Autodesk Inventor part; units mm, degrees
ref_plane "YZ Plane" through (0, 0, 0) normal (1, 0, 0) x (0, 1, 0)
ref_plane "XZ Plane" through (0, 0, 0) normal (0, 1, 0) x (-1, 0, 0)
ref_plane "XY Plane" through (0, 0, 0) normal (0, 0, 1) x (1, 0, 0)
sketch "Sketch1" plane through (0, 0, 0) normal (0, 1, 0) x (-1, 0, 0)
  line L0 (-10.795, 10.795) -> (10.795, 10.795)
  line L1 (10.795, 10.795) -> (10.795, -10.795)
  line L2 (-10.795, -10.795) -> (-10.795, 10.795)
  circle A0 centre (5.6576, -5.6576) radius 1.9304
  circle A1 centre (6.9088, 6.9088) radius 1.9304
  circle A2 centre (-5.6576, 5.6576) radius 1.9304
  circle A3 centre (-6.9088, -6.9148) radius 1.9304
  line L3 (-5.715, -10.795) -> (-5.715, -20.574)
  line L4 (-5.715, -20.574) -> (6.985, -20.574)
  line L5 (6.985, -20.574) -> (6.985, -10.795)
  line L6 (10.795, -10.795) -> (6.985, -10.795)
  line L7 (-5.715, -10.795) -> (-10.795, -10.795)
  point P0 (0, 0)
  dimension "d2" = 10.795
  dimension "d3" = 10.795
  dimension "d4" = 3.8608
  dimension "d5" = 5.6576
  dimension "d6" = 5.6576
  dimension "d7" = 3.8608
  dimension "d8" = 6.9088
  dimension "d9" = 6.9088
  dimension "d10" = 3.8608
  dimension "d11" = 5.6576
  dimension "d12" = 5.6576
  dimension "d13" = 3.8608
  dimension "d14" = 12.7
  dimension "d16" = 6.985
  dimension "d45" = 10.795
  dimension "d46" = 10.795
  dimension "d47" = 10.795
extrude "Extrusion1" add sketch "Sketch1" along normal blind 6.985
sketch "Sketch2" plane through (-6.985, 0, -20.574) normal (-1, 0, 0) x (0, 0, 1)
  circle A0 centre (5.08, 3.4925) radius 4.6609 construction
  line L0 (9.779, 0) -> (0, 0)
  line L1 (0, 0) -> (0, 6.985)
  line L2 (9.7409, 3.4925) -> (7.4105, -0.544)
  line L3 (7.4105, -0.544) -> (2.7496, -0.544)
  line L4 (2.7496, -0.544) -> (0.4191, 3.4925)
  line L5 (0.4191, 3.4925) -> (2.7495, 7.529)
  line L6 (2.7495, 7.529) -> (7.4104, 7.529)
  line L7 (7.4104, 7.529) -> (9.7409, 3.4925)
  point P0 (20.574, 0)
  dimension "d19" = 9.3218
  dimension "d20" = 3.4925
  dimension "d21" = 5.08
extrude "Extrusion2" cut sketch "Sketch2" against normal blind 3.81
sketch "Sketch3" plane through (5.715, 0, -10.795) normal (1, 0, 0) x (0, 0, -1)
  circle A0 centre (4.699, 3.4925) radius 1.9304
  line L0 (9.779, 0) -> (9.779, 6.985)
  line L1 (0, 6.985) -> (9.779, 6.985)
  point P0 (-10.795, 0)
  dimension "d24" = 3.8608
  dimension "d25" = 5.08
  dimension "d26" = 3.4925
extrude "Extrusion3" cut sketch "Sketch3" against normal through all
sketch "Sketch4" plane through (0, 6.985, 0) normal (0, 1, 0) x (1, 0, 0)
  circle A0 centre (0, 0) radius 4
  dimension "d29" = 8
extrude "Extrusion4" add sketch "Sketch4" along normal blind 12.7
sketch "Sketch5" plane through (0, 19.685, 0) normal (0, 1, 0) x (1, 0, 0)
  arc A0 (2.0472, -2.5908) -> (-2.0472, -2.5908) centre (0, 0) ccw
  line L0 (-2.0472, -2.5908) -> (2.0472, -2.5908)
  dimension "d32" = 6.604
  dimension "d33" = 2.5908
fillet "Fillet1" radius 3.3782 4 edges at (10.795, 3.4925, 10.795) (10.795, 3.4925, -10.795) (-10.795, 3.4925, 10.795) (-10.795, 3.4925, -10.795)
extrude "Extrusion5" cut sketch "Sketch5" against normal through all
sketch "Sketch6" plane through (0, 19.685, 0) normal (0, 1, 0) x (1, 0, 0)
  line L0 (-6.985, 20.574) -> (5.715, 20.574)
  line L1 (0.635, 0) -> (0.635, 20.574)
  line L2 (0.635, 20.574) -> (-0.635, 20.574)
  line L3 (-0.635, 20.574) -> (-0.635, 0)
  line L4 (-0.635, -20.574) -> (0.635, 20.574) construction
  line L5 (0.635, -20.574) -> (-0.635, 20.574) construction
  line L6 (-0.635, 0) -> (0.635, 0)
  point P0 (0, 0)
  dimension "d37" = 1.27
extrude "Extrusion6" cut sketch "Sketch6" against normal through all
sketch "Sketch7" plane through (0, 0, 0) normal (0, -1, 0) x (1, 0, 0)
  circle A0 centre (-5.6576, -5.6576) radius 1.9304
  circle A1 centre (-5.6576, -5.6576) radius 4.6609 construction
  circle A2 centre (5.6576, 5.6576) radius 1.9304
  circle A3 centre (5.6576, 5.6576) radius 4.6609 construction
  line L0 (-5.6576, -0.9967) -> (-1.6211, -3.3271)
  line L1 (-1.6211, -3.3271) -> (-1.6211, -7.988)
  line L2 (-1.6211, -7.988) -> (-5.6576, -10.3185)
  line L3 (-5.6576, -10.3185) -> (-9.694, -7.988)
  line L4 (-9.694, -7.988) -> (-9.694, -3.3271)
  line L5 (-9.694, -3.3271) -> (-5.6576, -0.9967)
  line L6 (5.6576, 0.9967) -> (1.6211, 3.3271)
  line L7 (1.6211, 3.3271) -> (1.6211, 7.988)
  line L8 (1.6211, 7.988) -> (5.6576, 10.3185)
  line L9 (5.6576, 10.3185) -> (9.694, 7.988)
  line L10 (9.694, 7.988) -> (9.694, 3.3271)
  line L11 (9.694, 3.3271) -> (5.6576, 0.9967)
  point P0 (0, 0)
  dimension "d40" = 9.3218
  dimension "d41" = 9.3218
extrude "Extrusion7" cut sketch "Sketch7" against normal blind 4.3688
fillet "Fillet2" radius 1.27 1 edges at (5.715, 3.4925, -20.574)
properties part number "clamping hub .25 in to 8mm hub"
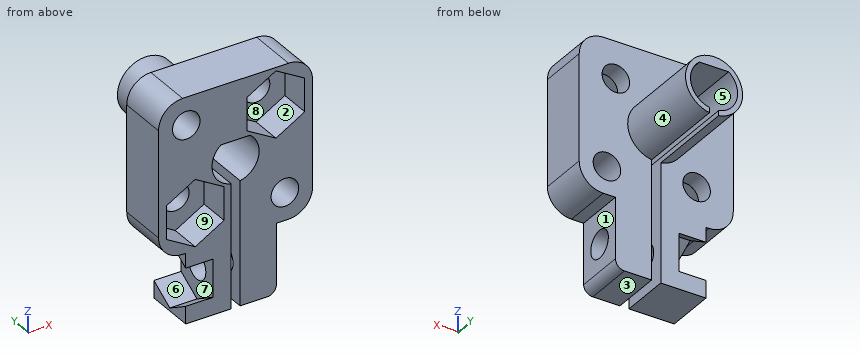
Here's how the part is built. I have some questions about the finished solid (model axes, mm). Face numbers are marked on the shaded views. A direction names the side the tool comes from. Give positions to 0.01 mm unless a question says otherwise; leave off trailing zeros. Loops run counter-clockwise (first coordinate to the right, second up) from the corner with the lowest first, then second, coordinate; pieces in that order, holes last. Notation, with made-up numbers: (87, -22.75) -> (135, -22.75) arc R8 cw to (135, -9.75) -> close; hole circle Ø11 at (81.5, 39.25). An arc over 180 degrees is marked (long way). Answer as a JSON object with one key per item and string values. Group by question number.
Item 1: I need wall thicknesses on L1, parallel to X at y = 2, z = -3.5 (3 decimals); L2, parallel to X at y = 2.25, z = 7 (3 decimals); L3, parallel to Y at x = 1.75, z = -7 (3 decimals). Which ranges of each line are inside material? Lowest first, please.
Item 2: Imagine slicing it at B-B on x = 8.25. Write out the boundary of the cut face in (y, z) (3 decimals).
Item 3: Imagine slicing it at C-C on z = -15.5. Write out the boundary of the cut face in (x, y) (3 decimals).
Item 4: Imagine slicing it at A-A on z = 0. Write out the boundary of the cut face in (x, y) (3 decimals), then the cut area to 3 significant figures.
Item 5: Imagine slicing it at D-D on x = 0. Write out the boundary of the cut face in (y, z) (3 decimals).
Item 6: On a 3-axis mill with a long thin cutter (end or side, diameter ignored), from which of +Z, -Z, +X, -X, +Y, -Y can I reach the whole of each face in a straight line? I mean the marked faces 1, 2, 3, 4 and 5. Say none if no direction works.
Item 7: Will these pins go through, and if not, where does the flat tip stop? pin 1 (1.5 mm diameter, centred on x = 2, z = -6, fed in from +Y) (3 decimals); pin 2 (3.5 mm diameter, centred on y = 3.5, z = -13.5, fed in from +X) (3 decimals); pin 3 (7.5 mm diameter, centred on y = 3.5, z = -13.5, fed in from -X).
Item 8: Thinking about a two-plate mould opening in Y: for the marked faces 6, 7, 8 and 9, which applies, pulls with the +Y half, pulls with the -Y half, needs draft (parallel to the pull), parting line crosses it, or undercut?
Answer list:
{
 "1": {"L1": "x = -10.795 to -9.694, -1.621 to -0.635, 0.635 to 10.795", "L2": "x = -10.795 to -8.837, -4.981 to 1.621, 9.694 to 10.795", "L3": "y = 0 to 6.985"},
 "2": {"outline": "(0, -10.691) -> (6.985, -10.691) -> (6.985, -8.303) -> (0, -8.303) -> close; (0, -5.526) -> (6.985, -5.526) -> (6.985, 10.691) -> (0, 10.691) -> (0, 8.822) -> (4.369, 8.822) -> (4.369, 2.493) -> (0, 2.493) -> close"},
 "3": {"outline": "(-3.175, 0) -> (-0.635, 0) -> (-0.635, 1.562) -> (-3.175, 1.562) -> close; (-3.175, 5.423) -> (-0.635, 5.423) -> (-0.635, 6.985) -> (-3.175, 6.985) -> close; (0.635, 0) -> (5.715, 0) -> (5.715, 1.562) -> (0.635, 1.562) -> close; (0.635, 5.423) -> (5.715, 5.423) -> (5.715, 6.985) -> (0.635, 6.985) -> close"},
 "4": {"outline": "(-10.795, 0) -> (-3.302, 0) -> (-3.302, 19.685) -> (-4, 19.685) -> (-4, 6.985) -> (-10.795, 6.985) -> close; (3.302, 0) -> (10.795, 0) -> (10.795, 6.985) -> (4, 6.985) -> (4, 19.685) -> (3.302, 19.685) -> close", "area": "122 mm2"},
 "5": {"outline": "(0, 2.591) -> (19.685, 2.591) -> (19.685, 4) -> (6.985, 4) -> (6.985, 10.795) -> (0, 10.795) -> close"},
 "6": {"face 1": "-Z, +X, +Y, -Y", "face 2": "-Y", "face 3": "-Z, +X, -X, +Y, -Y", "face 4": "+Y", "face 5": "+Y, -Y"},
 "7": {"pin 1": "stops at y = 6.985", "pin 2": "stops at x = 5.715", "pin 3": "stops at x = -9.86"},
 "8": {"face 6": "undercut", "face 7": "undercut", "face 8": "pulls with the -Y half", "face 9": "needs draft"}
}
